The listing builds one solid part. Answer for the finished solid, in the listing's coordinates (mm). Face numbers are marked on the shaded views. A direction names the side the tool comes from. Give positions to 0.01 mm unless a question says otherwise; leave off trailing zeros. Loops run counter-clockwise (first coordinate to the right, second up) from the corner with the lowest first, then second, coordinate; pieces in that order, holes last. Notation, with made-up numbers: (45, 27.5) - (59, 27.5) arc R20 ccw to (59, 42.5) - close; hole circle Ø11 at (-40, -1.5). An arc over 180 degrees is marked (long way). Answer in a Markdown table with one row per item. Add a question column.
```python
from build123d import *

# Parameters (mm, degrees)
F1_W     = 82.55
F1_H     = 82.55
F2_DEPTH = 41.275
F3_DEPTH = 82.55
F4_W     = 6.6821798682
F4_H     = 53.7756439298
F4_H_2   = 29.7516137362
F4_R     = 3.7333162537
F5_DEPTH = 67.31


# Not quite as in the source:
# - a variable given as a bare number and used for a length is read in inches; the dataset says mm whatever the document's units were


with BuildPart() as f2:
    # F1 (on Top) → F2 (new body, symmetric)
    with BuildSketch(Plane.XY):
        Rectangle(F1_W, F1_H)
    extrude(amount=F2_DEPTH, both=True)

    # F3 (add): a face of the model
    f3_faces = [f2.faces().sort_by_distance(p)[0] for p in [
        (41.275, 0, 0),
    ]]
    extrude(f3_faces, amount=F3_DEPTH)

    # F4 (on face) → F5 (join)
    with BuildSketch(Plane(origin=(0, 0, -41.275), x_dir=(1, 0, 0), z_dir=(0, 0, -1))):
        Polygon((117.642775178, -23.7058307976), (107.4604094028, -23.7058307976), (107.4604094028, 23.7058326602), (117.642775178, 23.7058326602), (117.642775178, 30.0698131323), (86.1410722136, 30.0698131323), (86.1410722136, 23.7058326602), (98.2326343656, 23.7058326602), (98.2326343656, -23.7058307976), (86.1410722136, -23.7058307976), (86.1410722136, -31.6608063877), (117.642775178, -31.6608063877), align=None)
        with Locations((77.0723931491, 3.1819911674)):
            Rectangle(F4_W, F4_H)
        with Locations((64.0262328088, 14.8758068681)):
            Rectangle(F4_W, F4_H_2)
        Polygon((60.6851428747, -10.9778670594), (67.3673227429, -11.2960664555), (67.3673227429, -3.9774877951), (60.6851428747, -3.9774877951), align=None)
        with BuildLine():
            Line((47.6389825344, 0), (53.3665642142, 0))
            Line((53.3665642142, 0), (53.3665642142, 29.7516137362))
            Line((53.3665642142, 29.7516137362), (47.6389825344, 29.7516137362))
            Line((47.6389825344, 29.7516137362), (39.7581494696, 8.1140771508))
            Line((39.7581494696, 8.1140771508), (33.0018214881, 30.0698131323))
            Line((33.0018214881, 30.0698131323), (33.0018214881, 4.0570385754))
            ThreePointArc((33.0018214881, 4.0570385754), (41.8631479069, 0.5195718098), (47.6389825344, 8.1140771508))
            Line((47.6389825344, 8.1140771508), (47.6389825344, 0))
        make_face()
        with BuildLine():
            ThreePointArc((7.5458958745, 29.43341434), (6.649165746, 16.0704833991), (11.6824880242, 3.6592902616))
            ThreePointArc((11.6824880242, 3.6592902616), (19.7418824044, 0.862989669), (28.2288361341, 0))
            Line((28.2288361341, 0), (28.2288361341, 6.8412809633))
            ThreePointArc((28.2288361341, 6.8412809633), (19.3054549337, 7.9595465035), (12.0006818324, 13.2052628323))
            ThreePointArc((12.0006818324, 13.2052628323), (21.7952321918, 15.7282111285), (25.9655225304, 24.9427194354))
            Line((25.9655225304, 24.9427194354), (25.8736382976, 29.1471914205))
            Line((25.8736382976, 29.1471914205), (7.5458958745, 29.43341434))
        make_face()
        with Locations((15.6531465528, 21.2212410615)):
            Circle(F4_R, mode=Mode.SUBTRACT)
    extrude(amount=F5_DEPTH)


solid = f2.part
```
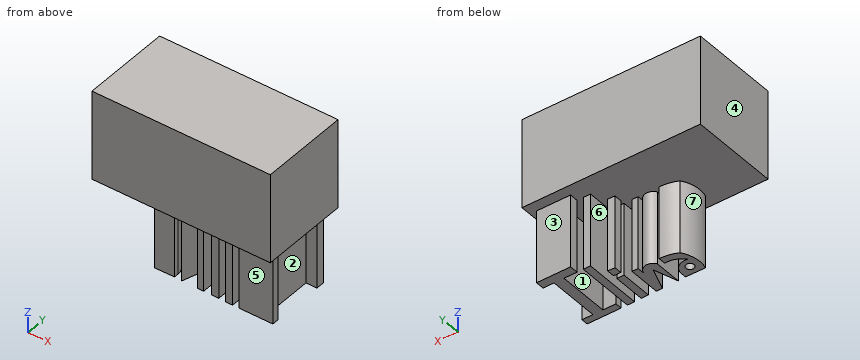
(1) Given pin 1 Ø6 at (x, z) = (17, -48) entering from -Y; pin 2 Ø5 at (x, z) = (113, -88.5) entering from +Y; pin 3 Ø5.5 at (y, z) = (7, -61) entering from -X, each flat-ended and moving along its own axis, determine where each tip first touches the part or whether it passes through.
(2) A cutting plane is placed at A-A on y = 9. Determine the outline of the cut face in (x, z) (3 decimals).
(3) The mould has two halves that part along X. Classify the marked faces 1, 2, 3 and 4: pulls with the +X half, pulls with the -X half, needs draft (parallel to the pull), parting line crosses it, or undercut.
(4) A cutting plane is placed at C-C on z = -70.5. Give the number of separate pieces and of enclosed holes in the cut face, plus the area to 3 significant figures.
(5) A cutting plane is placed at B-B on x = 90. Determine the outline of the cut face in (y, z) (3 decimals).
(6) A cutting plane is placed at D-D on y = -15.5. Determine the outline of the cut face in (x, z) (3 decimals), plus the area to 3 significant figures.
(7) Find the intervals of material crossed by line 1 along X through (y, z) = (-14.5, -51.5); line 2 along X through (y, z) = (11.5, -99); line 3 along X through (y, z) = (-10.5, -56.5), in increasing order. Write a range as [from, to].
(8) A tool of negligible diameter and unlimited length cuts with its end or side. For the marked faces 5, 6 and 7, from which of +Z, -Z, +X, -X, +Y, -Y can it reach the whole face along a straight path? Write none if from no direction.
Evaluation:
| question | item | result |
|---|---|---|
| 1 | pin 1 | stops at y = -29.33 |
| 1 | pin 2 | stops at y = 31.66 |
| 1 | pin 3 | stops at x = 60.69 |
| 2 | outline | (-41.275, -41.275) - (60.685, -41.275) - (60.685, -108.585) - (67.367, -108.585) - (67.367, -41.275) - (73.731, -41.275) - (73.731, -108.585) - (80.413, -108.585) - (80.413, -41.275) - (98.233, -41.275) - (98.233, -108.585) - (107.46, -108.585) - (107.46, -41.275) - (123.825, -41.275) - (123.825, 41.275) - (-41.275, 41.275) - close |
| 3 | face 1 | undercut |
| 3 | face 2 | pulls with the +X half |
| 3 | face 3 | needs draft |
| 3 | face 4 | pulls with the -X half |
| 4 | separate pieces | 6 |
| 4 | enclosed holes | 1 |
| 4 | area | 2,310 mm² |
| 5 | outline | (-41.275, -41.275) - (-30.07, -41.275) - (-30.07, -108.585) - (-23.706, -108.585) - (-23.706, -41.275) - (23.706, -41.275) - (23.706, -108.585) - (31.661, -108.585) - (31.661, -41.275) - (41.275, -41.275) - (41.275, 41.275) - (-41.275, 41.275) - close |
| 6 | outline | (-41.275, -41.275) - (6.746, -41.275) - (6.746, -108.585) - (21.515, -108.585) - (21.515, -41.275) - (33.002, -41.275) - (33.002, -108.585) - (37.485, -108.585) - (37.485, -41.275) - (42.448, -41.275) - (42.448, -108.585) - (53.367, -108.585) - (53.367, -41.275) - (60.685, -41.275) - (60.685, -108.585) - (67.367, -108.585) - (67.367, -41.275) - (73.731, -41.275) - (73.731, -108.585) - (80.413, -108.585) - (80.413, -41.275) - (98.233, -41.275) - (98.233, -108.585) - (107.46, -108.585) - (107.46, -41.275) - (123.825, -41.275) - (123.825, 41.275) - (-41.275, 41.275) - close |
| 6 | area | 17,200 mm² |
| 7 | line 1 | x = [6.94, 20.03], [33, 37.79], [42.08, 53.37], [60.69, 67.37], [73.73, 80.41], [98.23, 107.46] |
| 7 | line 2 | x = [73.73, 80.41], [98.23, 107.46] |
| 7 | line 3 | x = [8.11, 14.82], [33, 39.02], [40.63, 53.37], [60.69, 67.37], [73.73, 80.41], [98.23, 107.46] |
| 8 | face 5 | -Z, +X, -X, -Y |
| 8 | face 6 | -Z, +Y, -Y |
| 8 | face 7 | -Z, -X |
